The model under review builds one solid part; all positions refer to its coordinate system, in mm. Round coordinates to 2 decimals unless told otherwise and drop trailing zeros. Write each loop counter-clockwise with the first axis right and the second up, starting at its lowest first coordinate (ties: lowest second). Pieces come first, ordered by that corner, then holes. Notation, with made-up numbers: (29, 66) - (47, 66) arc R28 cw to (47, 91) - close; hole circle Ø6 at (39.5, 50.5). An arc over 180 degrees is marked (long way). Use one line per item in the form item = value.
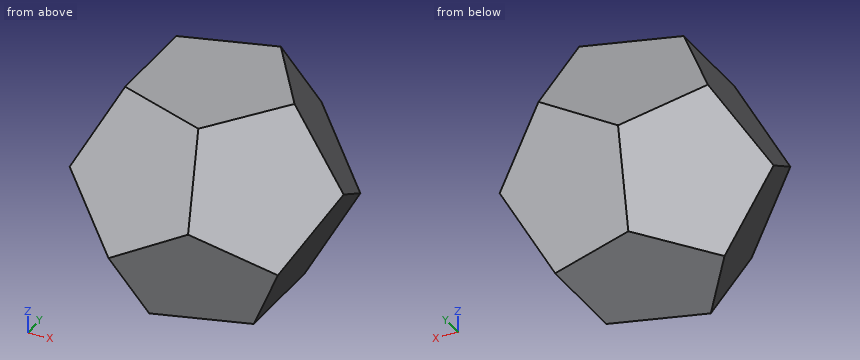
Solid Edge part; units mm, degrees
sketch "Sketch1" plane through (0, 0, 0) normal (0, -1, 0) x (1, 0, 0)
  line L0 (0, 151.7064) -> (0, -50.4015)
  arc A0 (0, 151.7065) -> (0, -50.4015) centre (0, 50.6525) cw
revolve "RevolvedProtrusion1" add sketch "Sketch1" angle 360 about axis through (0, 0, 151.7064) along (0, 0, -1)
sketch "Sketch2" plane through (0, 0, 0) normal (0, -1, 0) x (1, 0, 0)
  line L0 (62.6099, 62.6099) -> (31.305, 0)
  line L1 (31.305, 0) -> (-38.695, 0)
extrude "Cutout1" cut sketch "Sketch2" along normal mid plane 851.8671 material side at (47.0022, 0, 31.2826)
sketch "Sketch3" plane through (0, 0, 0) normal (0, -1, 0) x (1, 0, 0)
  line L0 (-31.305, 101.305) -> (38.695, 101.305)
  line L1 (-62.6099, 38.695) -> (-31.305, 101.305)
extrude "ExtrudedCutout_17" cut sketch "Sketch3" along normal mid plane 614.7236 material side at (3.695, 0, 101.355)
pattern_circular "Pattern1" count 5 over 360 about axis through (0, 0, 0) along (0, 0, 1) of "ExtrudedCutout_17", "Cutout1"
(1) Add section B-B on z = 25. Write out the cut boundary in (x, y).
Geometry results:
outline = (-54.15, 0) - (-16.73, -51.5) - (43.8, -31.83) - (43.8, 31.83) - (-16.73, 51.5) - close
(2) To check wall thickness, follow L1, parallel to Y at x = -23, z = 51; L2, parallel to Z at x = -29.5, y = 49; L3, parallel to Y at x = 35.5, z = 78. State the ranges of each line that lie inside material, in increasing order.
Geometry results:
L1 = -51.89 to 51.89
L2 = 42.73 to 52.48
L3 = -24.22 to 24.22
(3) Add section C-C on x = -15. Write out the cut boundary in (y, z) (3 decimals).
Geometry results:
outline = (-59.546, 41.382) - (-46.165, 15.931) - (-32.614, 0) - (32.614, 0) - (46.165, 15.931) - (59.546, 41.382) - (28.042, 101.305) - (-28.042, 101.305) - close
(4) Insertion check: P1, Ø5, axis at x = -20.5, z = 52, coming from the -Y side; P2, Ø6, axis at y = -5.5, z = 82.5, coming from the -X side; P3, Ø4, axis at x = -45, z = 10.5, coming from the -Y side. Each pin has a flat end and moves straight along its axis. Give the tip position at first contact, or say it passes through.
Geometry results:
P1 = -53.72
P2 = -42.21
P3 = -3.49
(5) Add section A-A on y = 28. Write out the cut boundary in (x, z) (3 decimals).
Geometry results:
outline = (-53.512, 56.891) - (-18.352, 0) - (15.13, 0) - (38.539, 14.467) - (53.512, 44.414) - (18.352, 101.305) - (-15.13, 101.305) - (-38.539, 86.838) - close
(6) Add section D-D on z = 85. Write out the cut boundary in (x, y), then the cut area to 3 significant figures.
Geometry results:
outline = (-39.46, -28.67) - (15.07, -46.39) - (48.77, 0) - (15.07, 46.39) - (-39.46, 28.67) - close
area = 5,660 mm2
